from build123d import *

# Parameters (mm, degrees)
SKETCH1_W           = 120
SKETCH1_H           = 120
BOSS_EXTRUDE1_DEPTH = 250
BOSS_EXTRUDE1_DRAFT = -3
SKETCH2_W           = 146.203889642
SKETCH2_H           = 146.203889642
BOSS_EXTRUDE2_DEPTH = 146.2
SKETCH3_R           = 60
BOSS_EXTRUDE3_DEPTH = 60


with BuildPart() as part:
    # Sketch1 → Boss-Extrude1 (with draft: the straight prism first)
    with BuildSketch(Plane(origin=(0, 0, 0), x_dir=(0, 0, -1), z_dir=(1, 0, 0))):
        Rectangle(SKETCH1_W, SKETCH1_H)
    extrude(amount=BOSS_EXTRUDE1_DEPTH)
    # Boss-Extrude1: the draft: its side faces are tilted about the plane it starts from
    boss_extrude1_sides = [part.faces().sort_by_distance(p)[0] for p in [
        (125, 0, 60),
        (125, -60, 0),
        (125, 0, -60),
        (125, 60, 0),
    ]]
    draft(boss_extrude1_sides, Plane(origin=(0, 0, 0), x_dir=(0, 0, -1), z_dir=(1, 0, 0)), BOSS_EXTRUDE1_DRAFT)

    # Sketch2 → Boss-Extrude2 (add)
    with BuildSketch(Plane(origin=(250, 0, 0), x_dir=(0, 0, -1), z_dir=(1, 0, 0))):
        Rectangle(SKETCH2_W, SKETCH2_H)
    extrude(amount=BOSS_EXTRUDE2_DEPTH)

    # Sketch3 → Boss-Extrude3 (add)
    with BuildSketch(Plane(origin=(0, 73.101944821, 0), x_dir=(1, 0, 0), z_dir=(0, 1, 0))):
        with Locations(Location((323.1, 0, 0), (0, 0, 90))):
            Circle(SKETCH3_R)
    extrude(amount=BOSS_EXTRUDE3_DEPTH)


solid = part.part
The model under review builds one solid part; all positions refer to its coordinate system, in mm. A direction names the side the tool comes from. Round coordinates to 2 decimals unless told otherwise and drop trailing zeros. Order: outer loops, then holes, each group sorted by start corner. A loop starts at its lowest first (then second) coordinate and runs counter-clockwise, first axis right, second up. Notation, with made-up numbers: (36, 59.5) - (68, 59.5) arc R20 cw to (68, 85.5) - close; hole circle Ø2 at (73, -37.75). An arc over 180 degrees is marked (long way). Use one line per item in the form item = value.
Q1. To check wall thickness, follow line 1 (Y direction, x = 336.5, z = -60.5); line 2 (Y direction, x = 25, z = -30.5); line 3 (Z direction, x = 197.5, y = 55). State the ranges of each line that lie inside material, in increasing order.
Response values:
line_1 = -73.1 to 73.1
line_2 = -61.31 to 61.31
line_3 = -70.35 to 70.35
Q2. Add section C-C on y = 30. Give the boundary of the cut face in (x, z), then the cut area to 3 significant figures.
Response values:
outline = (0, -60) - (250, -73.1) - (396.2, -73.1) - (396.2, 73.1) - (250, 73.1) - (0, 60) - close
area = 54,700 mm^2
Q3. Clearance check with flat-ended pins moving along their axes: P1, Ø4, axis at x = 276, y = 87.5, coming from the +Z side; P2, Ø5, axis at x = 104, z = -14, coming from the -Y side; P3, Ø1, axis at x = 93.5, z = -14, coming from the -Y side. State where each tip first meets the part, or that it passes through.
Response values:
P1 = 39.57
P2 = -65.58
P3 = -64.93
Q4. Tool access review of faces 1 (the cylindrical face through (381.673, 102.682, 13.007)), 2 (the flat face through (123.25, 66.46, 1.02)): name each direction out of +Z, -Z, +X, -X, +Y, -Y from which nothing blocks a thin tool from reaching the whole face with its end or side.
Response values:
face_1 = +Y
face_2 = +Z, -Z, -X, +Y
Q5. Add section D-D on x = 366.5. Give the boundary of the cut face in (y, z).
Response values:
outline = (-73.1, -73.1) - (73.1, -73.1) - (73.1, -41.43) - (133.1, -41.43) - (133.1, 41.43) - (73.1, 41.43) - (73.1, 73.1) - (-73.1, 73.1) - close
Q6. Add section B-B on z = 0. Give the boundary of the cut face in (x, y).
Response values:
outline = (0, -60) - (250, -73.1) - (396.2, -73.1) - (396.2, 73.1) - (383.1, 73.1) - (383.1, 133.1) - (263.1, 133.1) - (263.1, 73.1) - (250, 73.1) - (0, 60) - close
Q7. Add section A-A on x = 323.1. Give the boundary of the cut face in (y, z), then the cut area to 3 significant figures.
Response values:
outline = (-73.1, -73.1) - (73.1, -73.1) - (73.1, -60) - (133.1, -60) - (133.1, 60) - (73.1, 60) - (73.1, 73.1) - (-73.1, 73.1) - close
area = 28,600 mm^2
